Source: CAD feature listing. Evaluate the final solid. Frame: model axes, mm. A direction names the side the tool comes from. Give positions to 0.01 mm unless a question says otherwise; leave off trailing zeros. Loops run counter-clockwise (first coordinate to the right, second up) from the corner with the lowest first, then second, coordinate; pieces in that order, holes last. Notation, with made-up numbers: M 81.25,57.25 L 114.25,57.25 A5 cw 114.25,63.25 Z; hole C 25.25,68 d4. An arc over 180 degrees is marked long. Answer in a Markdown table with one row per item.
```python
from build123d import *
from build123d.topology import SkipClean

# Parameters (mm, degrees)
SKETCH1_R                = 1.5
BOSS_EXTRUDE1_DEPTH      = 2.5
BOSS_EXTRUDE2_DEPTH      = 1.8
BOSS_EXTRUDE2_DEPTH_BACK = 2.5
SKETCH2_R                = 4.5
SKETCH2_R_2              = 1.5
SKETCH4_R                = 2.5
CUT_EXTRUDE1_DEPTH       = 2
BOSS_EXTRUDE3_START      = 0.75
SKETCH5_R                = 4.5
SKETCH5_R_2              = 2.5
BOSS_EXTRUDE3_DEPTH      = 0.75
BOSS_EXTRUDE4_DEPTH      = 2.5
CUT_EXTRUDE2_REACH       = 80.314
SKETCH7_R                = 1.5
SKETCH7_W                = 7
SKETCH7_H                = 16.5
SKETCH7_W_2              = 16
SKETCH7_H_2              = 8
CUT_EXTRUDE3_REACH       = 82.041
SKETCH9_W                = 2.5
SKETCH9_H                = 22.388822383
BOSS_EXTRUDE5_DEPTH      = 12.5
FILLET1_R                = 4
FILLET2_R                = 1
FILLET3_R                = 4
CUT_EXTRUDE4_DEPTH       = 74.103052287
CUT_EXTRUDE4_DEPTH_BACK  = 74.103052287
SKETCH10_W               = 26.624352611
SKETCH10_H               = 48.524798022
CIRPATTERN1_START        = -34.45
CIRPATTERN1_DEPTH        = 2.5


# Read off the part's stored shape, not the designer's step: CirPattern1
with BuildPart() as part:
    # Sketch1 → Boss-Extrude1 (new body)
    with BuildSketch(Plane(origin=(0, 0, 0), x_dir=(0, 0, -1), z_dir=(1, 0, 0))):
        with BuildLine():
            Line((0, 12.5), (34.45, 12.5))
            Line((34.45, 12.5), (34.45, -12.5))
            Line((34.45, -12.5), (0, -12.5))
            ThreePointArc((0, -12.5), (-12.5, 0), (0, 12.5))
        make_face()
        Circle(SKETCH1_R, mode=Mode.SUBTRACT)
    extrude(amount=BOSS_EXTRUDE1_DEPTH)

    # Sketch2 → Boss-Extrude2 (add, two sides: drawn at the far end of the back side and taken through both)
    with BuildSketch(Plane.ZY.offset(-BOSS_EXTRUDE2_DEPTH_BACK)):
        Circle(SKETCH2_R)
        Circle(SKETCH2_R_2, mode=Mode.SUBTRACT)
    extrude(amount=BOSS_EXTRUDE2_DEPTH + BOSS_EXTRUDE2_DEPTH_BACK)

    # Sketch4 → Cut-Extrude1 (cut)
    with BuildSketch(Plane(origin=(2.5, 0, 0), x_dir=(0, 0, -1), z_dir=(1, 0, 0))):
        Circle(SKETCH4_R)
    extrude(amount=-CUT_EXTRUDE1_DEPTH, mode=Mode.SUBTRACT)

    # Sketch5 → Boss-Extrude3 (add)
    with SkipClean():  # the faces are left unmerged after this step: merging them gives an invalid solid
        with BuildSketch(Plane(origin=(2.5, 0, 0), x_dir=(0, 0, -1), z_dir=(1, 0, 0)).offset(BOSS_EXTRUDE3_START)):
            with Locations(Location((0, 0, 0), (0, 0, 180))):
                Circle(SKETCH5_R)
            Circle(SKETCH5_R_2, mode=Mode.SUBTRACT)
        extrude(amount=-BOSS_EXTRUDE3_DEPTH)

    # Sketch6 → Boss-Extrude4 (add)
    with SkipClean():  # the faces are left unmerged after this step: merging them gives an invalid solid
        with BuildSketch(Plane(origin=(0, 0, -34.45), x_dir=(-1, 0, 0), z_dir=(0, 0, -1))):
            Polygon((-8.812505246, 36.25), (53.321583376, 36.25), (53.321583376, -36.25), (6.25, -36.25), (-19.178416624, -36.25), (-19.178416624, 36.25), align=None)
        extrude(amount=-BOSS_EXTRUDE4_DEPTH)
    add(part.part.scale(1), mode=Mode.REPLACE)  # the faces are merged on a copy

    # Sketch7 → Cut-Extrude2 (cut, up to next)
    with BuildSketch(Plane.XY.offset(-31.95), mode=Mode.PRIVATE) as cut_extrude2_sk1:
        with Locations((11.678416624, -28.75)):
            Circle(SKETCH7_R)
    cut_extrude2_tool1 = extrude(cut_extrude2_sk1.sketch, amount=-CUT_EXTRUDE2_REACH, mode=Mode.PRIVATE) & part.part
    # Sketch7 → Cut-Extrude2 (cut, up to next)
    with BuildSketch(Plane.XY.offset(-31.95), mode=Mode.PRIVATE) as cut_extrude2_sk2:
        with Locations(Location((11.678416624, 28.75, 0), (0, 0, 180))):
            Circle(SKETCH7_R)
    cut_extrude2_tool2 = extrude(cut_extrude2_sk2.sketch, amount=-CUT_EXTRUDE2_REACH, mode=Mode.PRIVATE) & part.part
    # Sketch7 → Cut-Extrude2 (cut, up to next)
    with BuildSketch(Plane.XY.offset(-31.95), mode=Mode.PRIVATE) as cut_extrude2_sk3:
        with Locations((-45.821583376, 28.75)):
            Circle(SKETCH7_R)
    cut_extrude2_tool3 = extrude(cut_extrude2_sk3.sketch, amount=-CUT_EXTRUDE2_REACH, mode=Mode.PRIVATE) & part.part
    # Sketch7 → Cut-Extrude2 (cut, up to next)
    with BuildSketch(Plane.XY.offset(-31.95), mode=Mode.PRIVATE) as cut_extrude2_sk4:
        with Locations(Location((-45.821583376, -28.75, 0), (0, 0, 180))):
            Circle(SKETCH7_R)
    cut_extrude2_tool4 = extrude(cut_extrude2_sk4.sketch, amount=-CUT_EXTRUDE2_REACH, mode=Mode.PRIVATE) & part.part
    # Sketch7 → Cut-Extrude2 (cut, up to next)
    with BuildSketch(Plane.XY.offset(-31.95), mode=Mode.PRIVATE) as cut_extrude2_sk5:
        with Locations((-1.711858899, -11.632438111)):
            Rectangle(SKETCH7_W, SKETCH7_H)
    cut_extrude2_tool5 = extrude(cut_extrude2_sk5.sketch, amount=-CUT_EXTRUDE2_REACH, mode=Mode.PRIVATE) & part.part
    # Sketch7 → Cut-Extrude2 (cut, up to next)
    with BuildSketch(Plane.XY.offset(-31.95), mode=Mode.PRIVATE) as cut_extrude2_sk6:
        with Locations((-16.5, 0)):
            Rectangle(SKETCH7_W_2, SKETCH7_H_2)
    cut_extrude2_tool6 = extrude(cut_extrude2_sk6.sketch, amount=-CUT_EXTRUDE2_REACH, mode=Mode.PRIVATE) & part.part
    add(cut_extrude2_tool1.solids().sort_by_distance((11.678417, -28.75, -31.95))[0], mode=Mode.SUBTRACT)
    add(cut_extrude2_tool2.solids().sort_by_distance((11.678417, 28.75, -31.95))[0], mode=Mode.SUBTRACT)
    add(cut_extrude2_tool3.solids().sort_by_distance((-45.821583, 28.75, -31.95))[0], mode=Mode.SUBTRACT)
    add(cut_extrude2_tool4.solids().sort_by_distance((-45.821583, -28.75, -31.95))[0], mode=Mode.SUBTRACT)
    add(cut_extrude2_tool5.solids().sort_by_distance((-1.711859, -11.632438, -31.95))[0], mode=Mode.SUBTRACT)
    add(cut_extrude2_tool6.solids().sort_by_distance((-16.5, 0, -31.95))[0], mode=Mode.SUBTRACT)

    # Sketch9 → Cut-Extrude3 (cut, up to next)
    with BuildSketch(Plane.XZ.offset(12.5), mode=Mode.PRIVATE) as cut_extrude3_sk1:
        with Locations((1.25, -20.755588809)):
            Rectangle(SKETCH9_W, SKETCH9_H)
    cut_extrude3_tool1 = extrude(cut_extrude3_sk1.sketch, amount=-CUT_EXTRUDE3_REACH, mode=Mode.PRIVATE) & part.part
    add(cut_extrude3_tool1.solids().sort_by_distance((1.25, -12.5, -20.755589))[0], mode=Mode.SUBTRACT)


with BuildPart() as cut_extrude3_piece_1:
    # of the separate pieces the step leaves, piece 1, a body of its own (cut_extrude3_pieces)
    add(part.part.solids().sort_by_distance((-53.321583376, 36.25, -31.95))[0])



with BuildPart() as cut_extrude3_piece_2:
    # of the separate pieces the step leaves, piece 2, a body of its own (cut_extrude3_pieces)
    add(part.part.solids().sort_by_distance((0, 12.5, 0))[0])


with BuildPart() as cut_extrude3_piece_1_1:
    add(cut_extrude3_piece_1.part)

    add(cut_extrude3_piece_2.part)  # Boss-Extrude5 merges Cut-Extrude3 piece 2
    # Sketch8 → Boss-Extrude5 (add, symmetric)
    with BuildSketch(Plane(origin=(0, 0, 0), x_dir=(1, 0, 0), z_dir=(0, 1, 0))):
        with BuildLine():
            Line((13.243344962, 31.95), (10.743344962, 31.95))
            Line((10.743344962, 31.95), (10.743344962, 24.009277686))
            ThreePointArc((10.743344962, 24.009277686), (9.553562393, 20.771648442), (6.550447712, 19.074849133))
            ThreePointArc((6.550447712, 19.074849133), (1.858764487, 16.423986378), (0, 11.365927519))
            Line((0, 11.365927519), (0, 9.071657281))
            Line((0, 9.071657281), (2.5, 9.071657281))
            Line((2.5, 9.071657281), (2.5, 11.666723736))
            ThreePointArc((2.5, 11.666723736), (3.641866376, 14.847101848), (6.545921975, 16.574853229))
            ThreePointArc((6.545921975, 16.574853229), (11.35315475, 19.434889059), (13.243344962, 24.69953272))
            Line((13.243344962, 24.69953272), (13.243344962, 31.95))
        make_face()
    extrude(amount=BOSS_EXTRUDE5_DEPTH, both=True)

    # Fillet1
    fillet1_edges = [cut_extrude3_piece_1_1.edges().sort_by_distance(p)[0] for p in [
        (11.993344962, -12.5, -31.95),
        (13.243344962, 0, -31.95),
        (10.743344962, 0, -31.95),
        (11.993344962, 12.5, -31.95),
    ]]
    fillet(fillet1_edges, radius=FILLET1_R)

    # Fillet2
    fillet2_edges = [cut_extrude3_piece_1_1.edges().sort_by_distance(p)[0] for p in [
        (-5.211858899, -19.882438111, -33.2),
        (-5.211858899, -3.382438111, -33.2),
        (1.788141101, -3.382438111, -33.2),
        (1.788141101, -19.882438111, -33.2),
        (-8.5, 4, -33.2),
        (-8.5, -4, -33.2),
        (-24.5, -4, -33.2),
        (-24.5, 4, -33.2),
    ]]
    fillet(fillet2_edges, radius=FILLET2_R)

    # Fillet3
    fillet3_edges = [cut_extrude3_piece_1_1.edges().sort_by_distance(p)[0] for p in [
        (19.178416624, 36.25, -33.2),
        (-53.321583376, 36.25, -33.2),
        (-53.321583376, -36.25, -33.2),
        (19.178416624, -36.25, -33.2),
    ]]
    fillet(fillet3_edges, radius=FILLET3_R)

    # Sketch10 → Cut-Extrude4 (cut, two sides: drawn at the far end of the back side and taken through both)
    with BuildSketch(Plane(origin=(0, 0, 0), x_dir=(1, 0, 0), z_dir=(0, 1, 0)).offset(-CUT_EXTRUDE4_DEPTH_BACK)):
        with Locations((4.711977851, 7.687600989)):
            Rectangle(SKETCH10_W, SKETCH10_H)
    extrude(amount=CUT_EXTRUDE4_DEPTH + CUT_EXTRUDE4_DEPTH_BACK, mode=Mode.SUBTRACT)

    # CirPattern1 outline → CirPattern1 (cut)
    with BuildSketch(Plane.XY.offset(CIRPATTERN1_START)):
        with BuildLine():
            ThreePointArc((-28.931307853, 18.882438111), (-29.224201072, 19.589544892), (-29.931307853, 19.882438111))
            Line((-29.931307853, 19.882438111), (-34.931307853, 19.882438111))
            ThreePointArc((-34.931307853, 19.882438111), (-35.638414634, 19.589544892), (-35.931307853, 18.882438111))
            Line((-35.931307853, 18.882438111), (-35.931307853, 4.382438111))
            ThreePointArc((-35.931307853, 4.382438111), (-35.638414634, 3.67533133), (-34.931307853, 3.382438111))
            Line((-34.931307853, 3.382438111), (-29.931307853, 3.382438111))
            ThreePointArc((-29.931307853, 3.382438111), (-29.224201072, 3.67533133), (-28.931307853, 4.382438111))
            Line((-28.931307853, 4.382438111), (-28.931307853, 18.882438111))
        make_face()
    extrude(amount=CIRPATTERN1_DEPTH, mode=Mode.SUBTRACT)


solid = cut_extrude3_piece_1_1.part
```
Q1. Reachability of faces 1 (the flat face through (-24.5, 0, -33)), 2 (the flat face through (-18, 36.25, -33)) from +Z, -Z, +X, -X, +Y, -Y: full face, straight path, thin tool, end or side. Return the list, or none.
Values follow:
| item | result |
|---|---|
| face 1 | +Z, -Z |
| face 2 | +Z, -Z, +X, -X, +Y |
Q2. Section query C-C (x = -46). Output: boundary loops of the cut face in (y, z).
Values follow:
| item | result |
|---|---|
| outline | M -36.25,-34.45 L -30.24,-34.45 L -30.24,-31.95 L -36.25,-31.95 Z; M -27.26,-34.45 L 27.26,-34.45 L 27.26,-31.95 L -27.26,-31.95 Z; M 30.24,-34.45 L 36.25,-34.45 L 36.25,-31.95 L 30.24,-31.95 Z |
Q3. Section query D-D (z = -33.9). Give the number of separate pieces and of enclosed holes in the cut face, plus the area to 3 significant figures.
Values follow:
| item | result |
|---|---|
| separate pieces | 1 |
| enclosed holes | 7 |
| area | 4,860 mm^2 |
Q4. Mould query, pull axis Y, two halves, no side actions, for faces 3 (the flat face through (-17, -4, -33)), 4 (the cylindrical face through (-52.12, 35.11, -33.18)), 5 (the flat face through (-26, 1, -34.45)). Classes: +Y half, -Y half, draft (parallel to the pull), parting line (faces both ways), or undercut.
Values follow:
| item | result |
|---|---|
| face 3 | undercut |
| face 4 | +Y half |
| face 5 | draft |
Q5. Section query B-B (y = 18). Output: boundary loops of the cut face in (x, z).
Values follow:
| item | result |
|---|---|
| outline | M -53.32,-34.45 L -35.93,-34.45 L -35.93,-31.95 L -53.32,-31.95 Z; M -28.93,-34.45 L 19.18,-34.45 L 19.18,-31.95 L -28.93,-31.95 Z |
Q6. Contact query for flat-ended pins moving along their axis: pin 1 Ø4 at (x, y) = (-45.82, 28.75) entering from -Z; pin 2 Ø2.5 at (x, y) = (-45.82, -28.75) entering from +Z (3 decimals). Output: stop coordinate, or through.
Values follow:
| item | result |
|---|---|
| pin 1 | z = -34.45 |
| pin 2 | through |
Q7. Ray query, probe 1 along X at (y, z) = (-14, -34.1); probe 2 along Y at (x, z) = (-13, -33.2); probe 3 along Y at (x, z) = (-31.5, -33.45). Return the intervals inside material, ascending. Write a range as from..to.
Values follow:
| item | result |
|---|---|
| probe 1 | -53.32..-5.21, 1.79..19.18 |
| probe 2 | -36.25..-4, 4..36.25 |
| probe 3 | -36.25..3.38, 19.88..36.25 |
Q8. Section query A-A (y = 28.75). Output: boundary loops of the cut face in (x, z), plus the area to 3 significant figures.
Values follow:
| item | result |
|---|---|
| outline | M -53.32,-34.45 L -47.32,-34.45 L -47.32,-31.95 L -53.32,-31.95 Z; M -44.32,-34.45 L 10.18,-34.45 L 10.18,-31.95 L -44.32,-31.95 Z; M 13.18,-34.45 L 19.18,-34.45 L 19.18,-31.95 L 13.18,-31.95 Z |
| area | 166 mm^2 |
